```python
from build123d import *

# Parameters (mm, degrees)
F1_DEPTH = 200
F2_R     = 2
F3_DEPTH = 8.301
F6_DEPTH = 25
F9_DEPTH = 150


# Not quite as in the source:
# - a feature names something its author has since deleted; it is built from what else it names


with BuildPart() as f1:
    # F0 (on Front) → F1 (new body)
    with BuildSketch(Plane.XZ):
        with BuildLine():
            Line((7.7333916469, 0.7795584959), (6.65, 1.65))
            ThreePointArc((6.65, 1.65), (5.917766953, 3.417766953), (4.15, 4.15))
            Line((4.15, 4.15), (-4.15, 4.15))
            ThreePointArc((-4.15, 4.15), (-5.917766953, 3.417766953), (-6.65, 1.65))
            Line((-6.65, 1.65), (-7.7333916469, 0.7795584959))
            ThreePointArc((-7.7333916469, 0.7795584959), (-8.1070622196, 0), (-7.7333916469, -0.7795584959))
            Line((-7.7333916469, -0.7795584959), (-6.65, -1.65))
            Line((-6.65, -1.65), (-6.65, -4.15))
            Line((-6.65, -4.15), (-4.15, -4.15))
            Line((-4.15, -4.15), (4.15, -4.15))
            Line((4.15, -4.15), (6.65, -4.15))
            Line((6.65, -4.15), (6.65, -1.65))
            Line((6.65, -1.65), (7.7333916469, -0.7795584959))
            ThreePointArc((7.7333916469, -0.7795584959), (8.1070622196, 0), (7.7333916469, 0.7795584959))
        make_face()
        with BuildLine():
            ThreePointArc((5.15, -1.65), (4.8571067812, -2.3571067812), (4.15, -2.65))
            Line((4.15, -2.65), (-4.15, -2.65))
            ThreePointArc((-4.15, -2.65), (-4.8571067812, -2.3571067812), (-5.15, -1.65))
            Line((-5.15, -1.65), (-5.15, 1.65))
            ThreePointArc((-5.15, 1.65), (-4.8571067812, 2.3571067812), (-4.15, 2.65))
            Line((-4.15, 2.65), (4.15, 2.65))
            ThreePointArc((4.15, 2.65), (4.8571067812, 2.3571067812), (5.15, 1.65))
            Line((5.15, 1.65), (5.15, -1.65))
        make_face(mode=Mode.SUBTRACT)
        with BuildLine():
            Line((-4.15, -2.65), (4.15, -2.65))
            ThreePointArc((4.15, -2.65), (4.8571067812, -2.3571067812), (5.15, -1.65))
            Line((5.15, -1.65), (5.15, 1.65))
            ThreePointArc((5.15, 1.65), (4.8571067812, 2.3571067812), (4.15, 2.65))
            Line((4.15, 2.65), (-4.15, 2.65))
            ThreePointArc((-4.15, 2.65), (-4.8571067812, 2.3571067812), (-5.15, 1.65))
            Line((-5.15, 1.65), (-5.15, -1.65))
            ThreePointArc((-5.15, -1.65), (-4.8571067812, -2.3571067812), (-4.15, -2.65))
        make_face()
    extrude(amount=F1_DEPTH)

    # F2 (on face) → F3 (cut, through all)
    with BuildSketch(Plane.XY.offset(4.15)):
        with Locations((0, -5)):
            Circle(F2_R)
    extrude(amount=-F3_DEPTH, mode=Mode.SUBTRACT)

    # F5 (on offset) → F6 (cut)
    with BuildSketch(Plane.XY.offset(4.6)):
        with BuildLine():
            Line((8, -3.7011680724), (8, 3.7011680724))
            Line((8, 3.7011680724), (-8, 3.7011680724))
            Line((-8, 3.7011680724), (-8, -3.7011680724))
            ThreePointArc((-8, -3.7011680724), (0, -0.1482238292), (8, -3.7011680724))
        make_face()
    extrude(amount=-F6_DEPTH, mode=Mode.SUBTRACT)

    # F8 (on offset) → F9 (cut)
    with BuildSketch(Plane.XZ.offset(200)):
        Polygon((-5.1262229681, -2.646596171), (0, -2.646596171), (5.1262229681, -2.646596171), (5.1262229681, -0.6600963534), (4.3867812492, 4.353403829), (0, 4.353403829), (-4.3867812492, 4.353403829), (-5.1262229681, -0.6600963534), align=None)
    extrude(amount=-F9_DEPTH, mode=Mode.SUBTRACT)


solid = f1.part
```
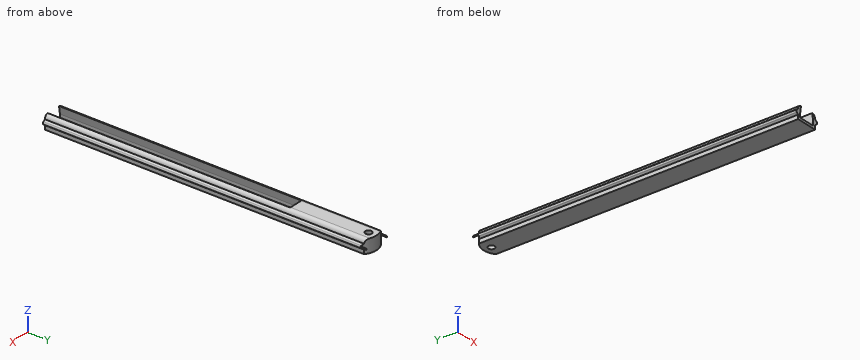
Geometry check sheet. Reference: the model listing, model coordinates, mm. Coordinates: 2 decimals unless noted, no trailing zeros. Order: outer loops, then holes, each group sorted by start corner. A loop starts at its lowest first (then second) coordinate and runs counter-clockwise, first axis right, second up. Notation, with made-up numbers: M -28,-6 L -22,-6 A24 cw -22,15 Z; hole C 35,-30 d2. An arc over 180 degrees is marked long. One line per question, with ' | ' between items. Start each with the question number.
Item 1: Cross-section at B-B on y = -186. Enter the section's corners in (x, z), then the cut area to 3 significant figures.
Item 2: Cross-section at A-A on x = 0. Enter the section's corners in (y, z).
Item 3: Gauge pin test, flat ends, axial feed: pin 1 (0.8 mm diameter, centred on y = -65.5, z = -2.5, fed in from +X); pin 2 (1 mm diameter, centred on y = -125, z = -1.5, fed in from +X); pin 3 (4 mm diameter, centred on x = 5.5, y = -106, fed in from +Z). Record the tip position at first contact, or that the pin passes through.
Item 4: Material ranges on L1, parallel to Y at x = 0, z = 1; L2, parallel to Y at x = 5.5, z = 1; L3, parallel to Z at x = -3.75, y = -115, recorded low to high. Write a range as [from, to].
Findings:
1) outline: M -7.73,-0.78 L -6.65,-1.65 L -6.65,-4.15 L 6.65,-4.15 L 6.65,-1.65 L 7.73,-0.78 A1 ccw 7.73,0.78 L 6.65,1.65 A2.5 ccw 4.42,4.14 L 5.13,-0.66 L 5.13,-2.65 L -5.13,-2.65 L -5.13,-0.66 L -4.42,4.14 A2.5 ccw -6.65,1.65 L -7.73,0.78 A1 ccw Z | area: 47.5 mm²
2) outline: M -200,-4.15 L -7,-4.15 L -7,4.15 L -50,4.15 L -50,-2.65 L -200,-2.65 Z; M -3,-4.15 L -0.15,-4.15 L -0.15,4.15 L -3,4.15 Z
3) pin 1: stops at x = 6.65 | pin 2: stops at x = 7.46 | pin 3: stops at z = 4.14
4) L1: y = [-50, -7], [-3, -0.15] | L2: y = [-200, -1.66] | L3: z = [-4.15, -2.65]
